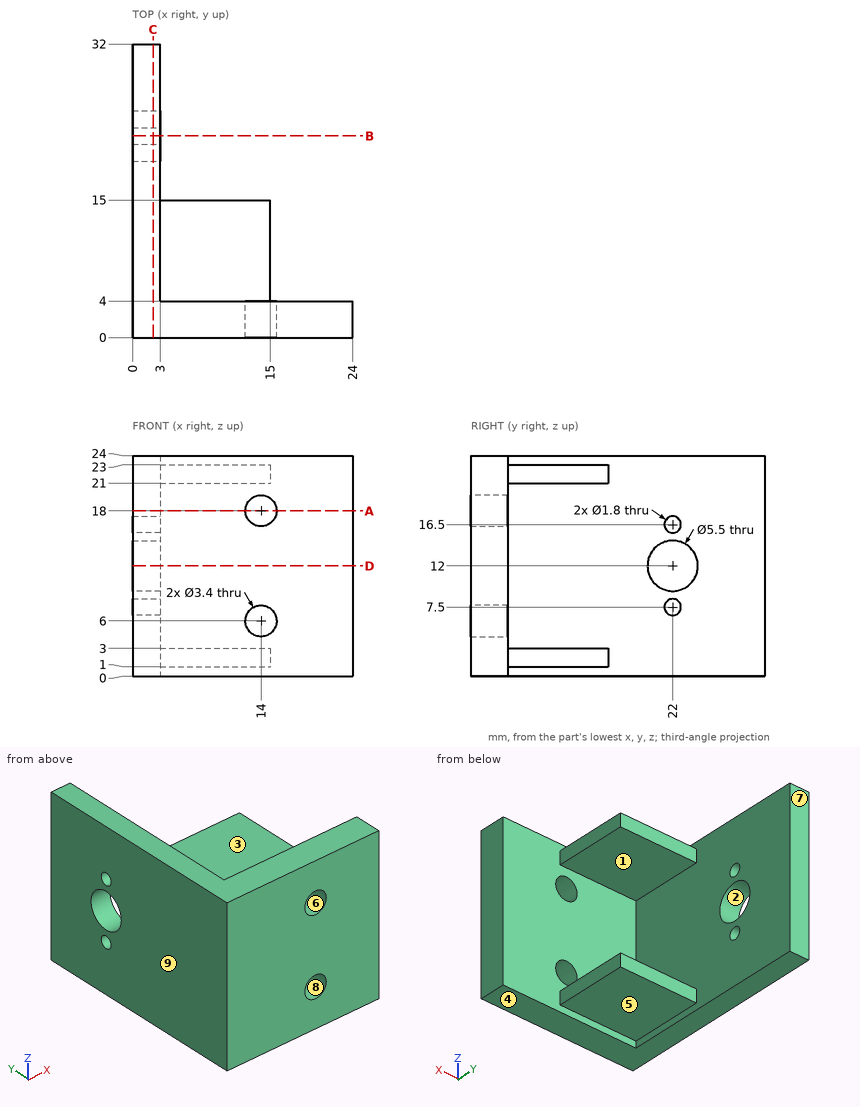
Can you work these out from the drawing? Everything is in mm from the part's minimum corner. A direction names the side the tool comes from. Give positions to 0.01 mm unless a question says otherwise; leave off trailing zeros. Loops run counter-clockwise (first coordinate to the right, second up) from the corner with the lowest first, then second, coordinate; pieces in that order, holes last. Notation, with made-up numbers: (80, 15) -> (99, 15) arc R22 ccw to (99, 38) -> close; hole circle Ø3 at (-15, 26.25). An arc over 180 degrees is marked (long way). Return JSON: item names as keys, results as strings.
Q1. On a 3-axis mill with a long thin cutter (end or side, diameter ignored), from which of +Z, -Z, +X, -X, +Y, -Y can I reach the whole of each face in a straight line? I mean the marked faces 1, 2, 3, 4 and 5. Say none if no direction works.
Checks:
{"face 1": "+X, +Y", "face 2": "+X, -X", "face 3": "+Z, +X, +Y", "face 4": "-Z, +X, -X, +Y, -Y", "face 5": "-Z, +X, +Y"}
Q2. I need wall thicknesses on probe 1 along Y at (x, z) = (2.2, 7.5); probe 2 along Z at (x, y) = (9.5, 13.5); probe 3 along Y at (x, z) = (20, 17.25). Which ranges of each line are inside material? Lowest first, please.
Checks:
{"probe 1": "y = 0 to 21.1, 22.9 to 32", "probe 2": "z = 1 to 3, 21 to 23", "probe 3": "y = 0 to 4"}
Q3. I want a section at C-C, the plane x = 2.25. List the corners of the cut face in (y, z) for me.
Checks:
{"outline": "(0, 0) -> (32, 0) -> (32, 24) -> (0, 24) -> close; hole circle Ø5.5 at (22, 12); hole circle Ø1.8 at (22, 7.5); hole circle Ø1.8 at (22, 16.5)"}
Q4. I want a section at A-A, the plane z = 18. List the corners of the cut face in (x, y) for me.
Checks:
{"outline": "(0, 0) -> (12.3, 0) -> (12.3, 4) -> (3, 4) -> (3, 32) -> (0, 32) -> close; (15.7, 0) -> (24, 0) -> (24, 4) -> (15.7, 4) -> close"}
Q5. I want a section at B-B, the plane y = 22. List the corners of the cut face in (x, z) for me, then the cut area to 3 significant figures.
Checks:
{"outline": "(0, 0) -> (3, 0) -> (3, 6.6) -> (0, 6.6) -> close; (0, 8.4) -> (3, 8.4) -> (3, 9.25) -> (0, 9.25) -> close; (0, 14.75) -> (3, 14.75) -> (3, 15.6) -> (0, 15.6) -> close; (0, 17.4) -> (3, 17.4) -> (3, 24) -> (0, 24) -> close", "area": "44.7 mm2"}
Q6. We'd pull the mould along X, two halves only. Please class the marked faces 6, 7, 8 and 9: released by +X, released by -X, zero draft, split by the parting line, or undercut.
Checks:
{"face 6": "undercut", "face 7": "zero draft", "face 8": "undercut", "face 9": "released by -X"}
Q7. For pin 1 Ø0.6 at (x, z) = (8.5, 2) entering from +Y; pin 2 Ø3 at (x, z) = (14, 6) entering from -Y; pin 3 Ø4.5 at (x, z) = (14, 18) entering from -Y; pin 4 Ø2 at (x, z) = (18, 14.5) entering from +Y, each with a flat end and sliding along its axis, tell me the tip position at first contact or that it passes through.
Checks:
{"pin 1": "stops at y = 15", "pin 2": "passes through", "pin 3": "stops at y = 0", "pin 4": "stops at y = 4"}
Q8. I want a section at D-D, the plane z = 12. List the corners of the cut face in (x, y) for me, then the cut area to 4 significant figures.
Checks:
{"outline": "(0, 0) -> (24, 0) -> (24, 4) -> (3, 4) -> (3, 19.25) -> (0, 19.25) -> close; (0, 24.75) -> (3, 24.75) -> (3, 32) -> (0, 32) -> close", "area": "163.5 mm2"}
